The figure shows three views and two pictorial views of one solid part (mm, origin at its lowest corner). Answer the questions. A direction names the side the tool comes from. Coordinates: 2 decimals unless noted, no trailing zeros. Order: outer loops, then holes, each group sorted by start corner. A loop starts at its lowest first (then second) coordinate and runs counter-clockwise, first axis right, second up. Notation, with made-up numbers: M 53,87 L 66,87 A25 cw 66,101 Z; hole C 35,35 d4. An arc over 180 degrees is marked long. Answer in a Markdown table with one row per item. Add a question column.
Item 1: The part is cut by section C-C (x = 50). Write down the section's boundary in (y, z).
Item 2: The part is cut by section D-D (x = 30). Write down the section's boundary in (y, z), then the cut area to 3 significant figures.
Item 3: Consider line 1 (X direction, y = 1, z = 40); line 2 (Y direction, x = 37.5, z = 11); line 3 (Z direction, x = 34, y = 33.5). Determine where each line is inside the solid, lowest interval first. Write a range as from..to.
Item 4: Flat-ended cylindrical pins translate along their axes: pin 1 Ø5 at (x, z) = (10, 40) entering from +Y; pin 2 Ø4 at (x, z) = (10, 10) entering from +Y; pin 3 Ø6 at (x, y) = (11.5, 28) entering from -Z; pin 4 Ø1 at (x, z) = (48, 36) entering from -Y. Find the tip coordinate at first contact, or state that the pin passes through.
Item 5: Which of the six approach directions +Z, -Z, +X, -X, +Y, -Y give full straight-line access (tool end or side, diameter ignored) to the marked faces 1, 2, 3 and 4?
Item 6: The part is cut by section A-A (z = 10). Write down the section's boundary in (x, y), then the cut area to 3 significant figures.
Item 7: The part is cut by section B-B (y = 86.5). Write down the section's boundary in (x, z).
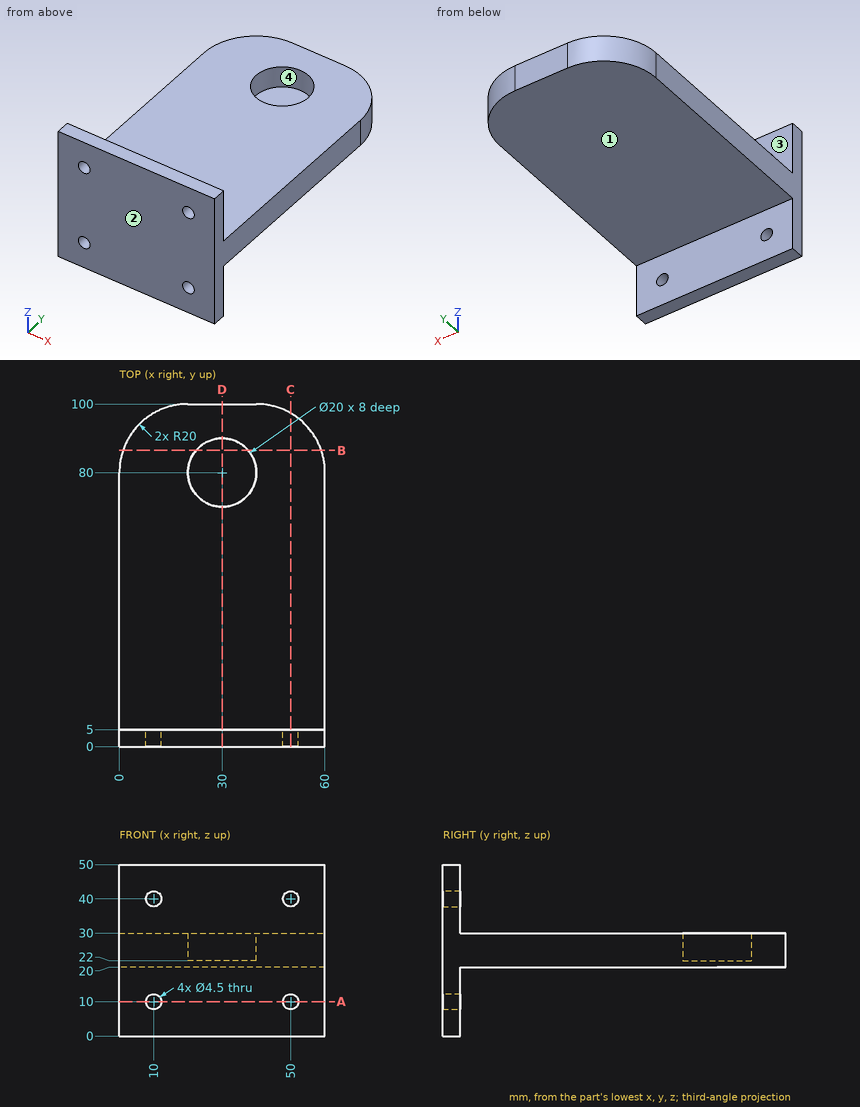
Reply:
| question | item | result |
|---|---|---|
| 1 | outline | M 0,0 L 5,0 L 5,7.75 L 0,7.75 Z; M 0,12.25 L 5,12.25 L 5,20 L 97.32,20 L 97.32,30 L 5,30 L 5,37.75 L 0,37.75 Z; M 0,42.25 L 5,42.25 L 5,50 L 0,50 Z |
| 2 | outline | M 0,0 L 5,0 L 5,20 L 100,20 L 100,30 L 90,30 L 90,22 L 70,22 L 70,30 L 5,30 L 5,50 L 0,50 Z |
| 2 | area | 1,040 mm2 |
| 3 | line 1 | x = 0..7.75, 12.25..47.75, 52.25..60 |
| 3 | line 2 | y = 0..5 |
| 3 | line 3 | z = 20..30 |
| 4 | pin 1 | stops at y = 5 |
| 4 | pin 2 | passes through |
| 4 | pin 3 | stops at z = 20 |
| 4 | pin 4 | stops at y = 0 |
| 5 | face 1 | -Z, +X, -X, +Y |
| 5 | face 2 | +Z, -Z, +X, -X, -Y |
| 5 | face 3 | +Z, +X, -X, +Y |
| 5 | face 4 | +Z |
| 6 | outline | M 0,0 L 7.75,0 L 7.75,5 L 0,5 Z; M 12.25,0 L 47.75,0 L 47.75,5 L 12.25,5 Z; M 52.25,0 L 60,0 L 60,5 L 52.25,5 Z |
| 6 | area | 255 mm2 |
| 7 | outline | M 1.09,20 L 58.91,20 L 58.91,30 L 37.6,30 L 37.6,22 L 22.4,22 L 22.4,30 L 1.09,30 Z |
